Study the drawing (mm; zero at the part's minimum x, y, z) and answer. Coordinates: 2 decimals unless noted, no trailing zeros. Loops run counter-clockwise (first coordinate to the right, second up) from the corner with the lowest first, then second, coordinate; pieces in that order, holes last. Notation, with made-up numbers: (20, 32.25) -> (68, 32.25) arc R30 ccw to (68, 59.25) -> close; hole circle Ø1 at (71, 33.25). An arc over 180 degrees is marked (long way). Answer as CSV lines item,"result".
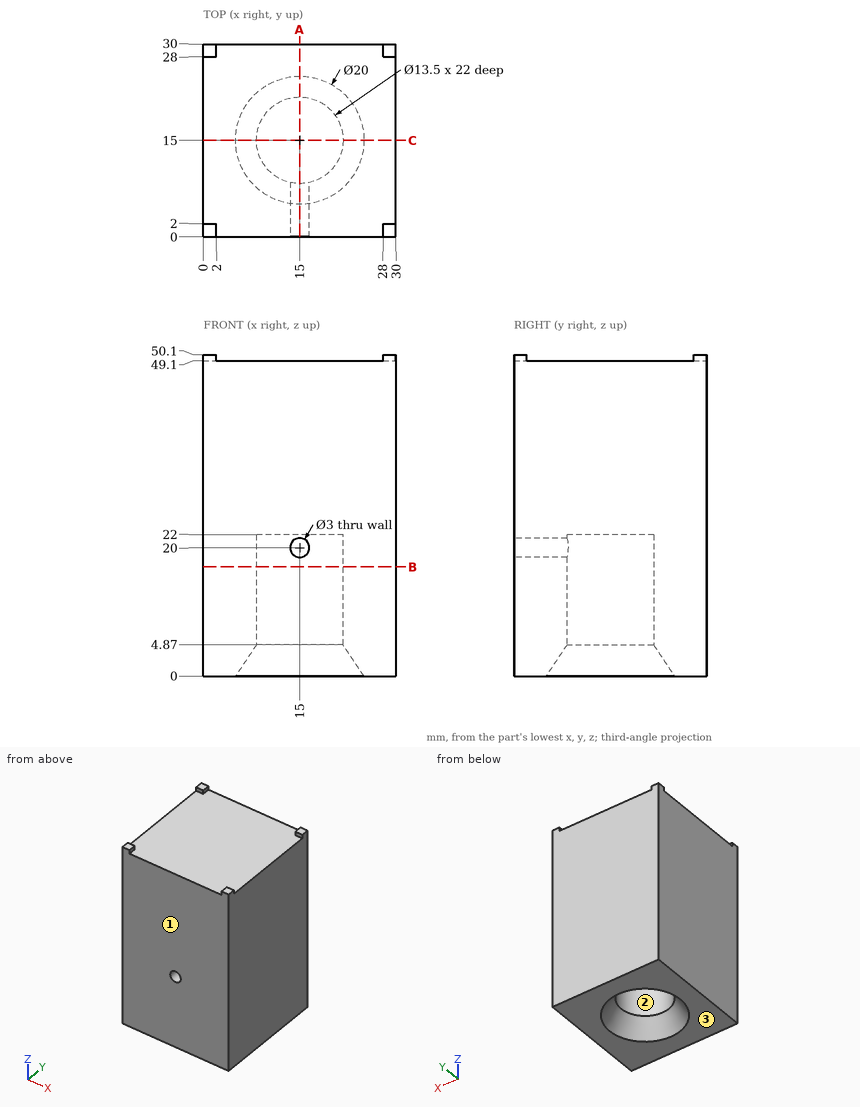
Q1. Given pin 1 Ø12 at (x, y) = (15, 15) entering from +Z; pin 2 Ø11 at (x, y) = (12, 14) entering from -Z (1 decimal), each flat-ended and moving along its own axis, determine where each tip first touches the part or whether it passes through.
Results:
pin 1,"stops at z = 49.1"
pin 2,"stops at z = 2"
Q2. Find the intervals of material crossed by probe 1 along Z at (x, y) = (15, 2.5); probe 2 along Y at (x, z) = (15, 13.75); probe 3 along X at (y, z) = (6.5, 20), in increasing order. Write a range as [from, to].
Results:
probe 1,"z = [0, 18.5], [21.5, 49.1]"
probe 2,"y = [0, 8.25], [21.75, 30]"
probe 3,"x = [0, 13.5], [16.5, 30]"
Q3. A cutting plane is placed at B-B, the plane z = 17. Write down the section's boundary in (x, y), and give its area (3 significant figures).
Results:
outline,"(0, 0) -> (30, 0) -> (30, 30) -> (0, 30) -> close; hole circle Ø13.5 at (15, 15)"
area,"757 mm²"
Q4. A cutting plane is placed at C-C, the plane y = 15. Write down the section's boundary in (x, z), and give its area (3 significant figures).
Results:
outline,"(0, 0) -> (5, 0) -> (8.25, 4.87) -> (8.25, 22) -> (21.75, 22) -> (21.75, 4.87) -> (25, 0) -> (30, 0) -> (30, 49.1) -> (0, 49.1) -> close"
area,"1,160 mm²"
Q5. For a pull along Y with two mould halves and no side action, classify the marked faces 1, 2 and 3 as pulls with the +Y half, pulls with the -Y half, needs draft (parallel to the pull), parting line crosses it, or undercut.
Results:
face 1,"pulls with the -Y half"
face 2,"undercut"
face 3,"needs draft"
Q6. A cutting plane is placed at A-A, the plane x = 15. Write down the section's boundary in (y, z), and give its area (3 significant figures).
Results:
outline,"(0, 0) -> (5, 0) -> (8.25, 4.87) -> (8.25, 18.5) -> (0, 18.5) -> close; (0, 21.5) -> (8.25, 21.5) -> (8.25, 22) -> (21.75, 22) -> (21.75, 4.87) -> (25, 0) -> (30, 0) -> (30, 49.1) -> (0, 49.1) -> close"
area,"1,140 mm²"
